Work out the finished part from the listing and answer in its coordinate system (mm). Face numbers are marked on the shaded views. A direction names the side the tool comes from. Round coordinates to 2 decimals unless told otherwise and drop trailing zeros. Order: outer loops, then holes, each group sorted by start corner. A loop starts at its lowest first (then second) coordinate and runs counter-clockwise, first axis right, second up. Notation, with made-up numbers: (-33.5, -6) -> (-19.5, -6) arc R19 ccw to (-19.5, 7) -> close; hole circle Ø1 at (-35, 45). An arc over 180 degrees is marked (long way). Use one line per item in the form item = value.
Autodesk Inventor part; units mm, degrees
ref_plane "YZ Plane" through (0, 0, 0) normal (1, 0, 0) x (0, 1, 0)
ref_plane "XZ Plane" through (0, 0, 0) normal (0, 1, 0) x (-1, 0, 0)
ref_plane "XY Plane" through (0, 0, 0) normal (0, 0, 1) x (1, 0, 0)
sketch "Náčrt1" plane through (0, 0, 0) normal (0, 0, 1) x (1, 0, 0)
  line L0 (0, 0) -> (-120, 0)
  line L1 (-120, 0) -> (-120, 11)
  line L2 (-120, 11) -> (-20.578, 11)
  line L3 (-20.578, 11) -> (-12, 15)
  line L4 (-12, 15) -> (0, 15)
  line L5 (0, 15) -> (0, 0)
  dimension "d2" = 22
  dimension "d3" = 30
  dimension "d4" = 12
  dimension "d5" = 25
  dimension "d6" = 120
revolve "Rotace1" add sketch "Náčrt1" angle 360 about axis through (0, 0, 0) along (-1, 0, 0)
hole "Díra1" at (0, 0, 0) direction (-1, 0, 0) diameter 22.38 depth 14 tip angle 118
hole "Díra2" at (0, 0, 0) direction (-1, 0, 0) diameter 19.2 depth 75 tip angle 118
hole "Díra3" at (-120, 0, 0) direction (1, 0, 0) diameter 8.92 depth 12 tip angle 118
chamfer "Zkosení1" distance 6 angle 30 1 edges at (-120, -11, 0) measured on face at (-53.7187, 10.8576, 1.7645)
sketch "Náčrt2" plane through (0, 0, 0) normal (1, 0, 0) x (0, 0, -1)
  circle A0 centre (16, 0) radius 2.6
  point P0 (0, 0)
  dimension "d40" = 16
  dimension "d41" = 5.2
extrude "Vysunutí1" cut sketch "Náčrt2" against normal blind 5
pattern_circular "Kruhové pole1" count 18 over 360 about axis through (-6, 0, 0) along (1, 0, 0) of "Vysunutí1"
chamfer "Zkosení2" distance 0.5 angle 45 1 edges at (0, 0, 11.19)
properties part number "Head03" material "ETG 100"
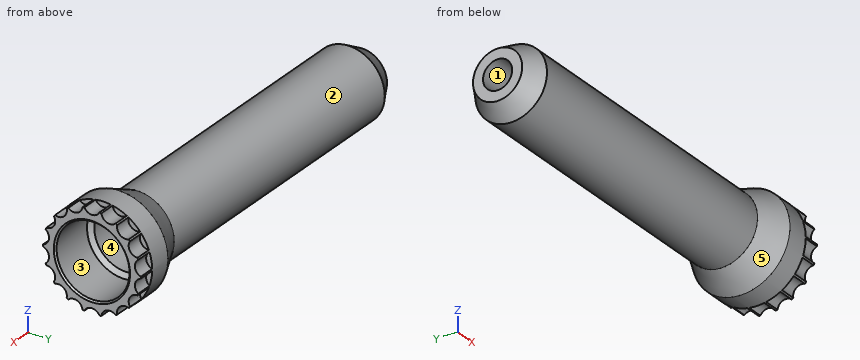
Item 1: The part is cut by section B-B, the plane x = -93.5. Give the vertices of the cut face in (y, z).
Findings:
outline = circle Ø22 at (0, 0)
Item 2: Consider line 1 along Z through (x, y) = (-113.75, 0); line 2 along Z through (x, y) = (-8, 0); line 3 along X through (y, z) = (8.5, -12.25). Determine where each line is inside the solid, lowest interval first.
Findings:
line_1 = -11 to -4.46, 4.46 to 11
line_2 = -15 to -11.19, 11.19 to 15
line_3 = -12.19 to -5
Item 3: For the marked faces 4 and 5, determine the directions among +Z, -Z, +X, -X, +Y, -Y from which every point of the face is accessible in a straight line to the end or side of a thin tool.
Findings:
face_4 = +X
face_5 = -X
Item 4: Determine the mould class of the marked faces 1, 2 and 3 for opening direction Y: released by +Y, released by -Y, zero draft, split by the parting line, or undercut.
Findings:
face_1 = undercut
face_2 = split by the parting line
face_3 = undercut
Item 5: Flat-ended cylindrical pins translate along their axes: P1, Ø11.5, axis at y = 0, z = 0, coming from the -X side; P2, Ø6, axis at x = -76, y = -9, coming from the +Z side; P3, Ø1.1, axis at y = 5, z = -14, coming from the +X side; P4, Ø3, axis at x = -51.5, y = -1, coming from the -Z side. Find the tip coordinate at first contact, or state that the pin passes through.
Findings:
P1 = -120
P2 = 9.22
P3 = -5
P4 = -11
Item 6: The part is cut by section A-A, the plane x = -60. Give the vertices of the cut face in (y, z), and give its area (3 significant figures).
Findings:
outline = circle Ø22 at (0, 0); hole circle Ø19.2 at (0, 0)
area = 90.6 mm^2
